Work out the finished part from the listing and answer in its coordinate system (mm). Face numbers are marked on the shaded views. A direction names the side the tool comes from. Round coordinates to 2 decimals unless told otherwise and drop trailing zeros. Loops run counter-clockwise (first coordinate to the right, second up) from the corner with the lowest first, then second, coordinate; pieces in that order, holes last.
```python
from build123d import *

# Parameters (mm, degrees)
F0_W     = 86.91734
F0_H     = 55.834315
F1_DEPTH = 25.4
F2_DEPTH = 25.4
F3_W     = 30.795218
F3_H     = 99.005182
F4_DEPTH = 25.4


with BuildPart() as f1:
    # F0 (on Front) → F1 (new body)
    with BuildSketch(Plane.XZ):
        with Locations((5.0366, -8.202463)):
            Rectangle(F0_W, F0_H)
    extrude(amount=F1_DEPTH)

    # F0 (on Front) → F2 (join)
    with BuildSketch(Plane.XZ):
        with Locations((5.0366, -8.202463)):
            Rectangle(F0_W, F0_H)
    extrude(amount=F2_DEPTH)

    # F3 (on Front) → F4 (join)
    with BuildSketch(Plane.XZ):
        with Locations((-0.287806, -13.958579)):
            Rectangle(F3_W, F3_H)
    extrude(amount=F4_DEPTH)


solid = f1.part
```
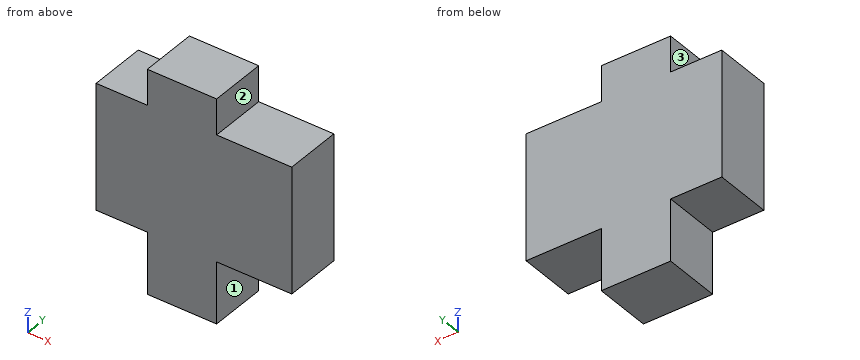
1. Find section A-A (y = -17). Write down the section's boundary in (x, z).
Answer key:
outline: (-38.42, -36.12) - (-15.69, -36.12) - (-15.69, -63.46) - (15.11, -63.46) - (15.11, -36.12) - (48.5, -36.12) - (48.5, 19.71) - (15.11, 19.71) - (15.11, 35.54) - (-15.69, 35.54) - (-15.69, 19.71) - (-38.42, 19.71) - close
2. Which of the six approach directions +Z, -Z, +X, -X, +Y, -Y give full straight-line access (tool end or side, diameter ignored) to the marked faces 1, 2 and 3?
Answer key:
face 1: -Z, +X, +Y, -Y
face 2: +Z, +X, +Y, -Y
face 3: +Z, -X, +Y, -Y
3. Find section C-C (x = -30). Write down the section's boundary in (y, z), then the cut area to 3 significant figures.
Answer key:
outline: (-25.4, -36.12) - (0, -36.12) - (0, 19.71) - (-25.4, 19.71) - close
area: 1,420 mm2
4. Given pin 1 (4.5 mm diameter, centred on y = -18.5, z = 26, fed in from +X); pin 2 (8 mm diameter, centred on x = 22.5, y = -3, fed in from -Z); pin 3 (7.5 mm diameter, centred on x = 33, y = -17.5, fed in from +Z); pin 4 (6 mm diameter, centred on y = -8.5, z = 22, fed in from +X), each flat-ended and moving along its own axis, determine where each tip first touches the part or whether it passes through.
Answer key:
pin 1: stops at x = 15.11
pin 2: stops at z = -36.12
pin 3: stops at z = 19.71
pin 4: stops at x = 48.5
5. Find section B-B (z = -39). Write down the section's boundary in (x, y).
Answer key:
outline: (-15.69, -25.4) - (15.11, -25.4) - (15.11, 0) - (-15.69, 0) - close
6. Consider probe 1 along Z at (x, y) = (-21, -16.75); probe 2 along X at (y, z) = (-7, -40). Determine where each line is inside the solid, lowest interval first.
Answer key:
probe 1: z = -36.12 to 19.71
probe 2: x = -15.69 to 15.11
